The model under review builds one solid part; all positions refer to its coordinate system, in mm. A direction names the side the tool comes from. Coordinates: 2 decimals unless noted, no trailing zeros. Write each loop counter-clockwise with the first axis right and the second up, starting at its lowest first coordinate (ties: lowest second). Pieces come first, ordered by that corner, then holes. Notation, with made-up numbers: (6.5, 49.5) - (22.5, 49.5) arc R9 cw to (22.5, 62.5) - close; hole circle Ø4 at (9, 24.25). An arc over 180 degrees is marked (long way). Use one line per item in the form item = value. Start each with the question number.
```python
from build123d import *
from OCP.BRepFilletAPI import BRepFilletAPI_MakeFillet

# Parameters (mm, degrees)
SKETCH_1_R      = 1.54
EXTRUDE_1_DEPTH = 5
SKETCH_2_R      = 1.7
EXTRUDE_2_DEPTH = 5
FILLET_1_R1     = 3
FILLET_1_R2     = 8


with BuildPart() as part:
    # 草图1 → 凸台-拉伸1 (new body)
    with BuildSketch(Plane.XY):
        with BuildLine():
            Line((0, -28.5), (76.583465403, -28.5))
            Line((76.583465403, -28.5), (76.583465403, 28.5))
            Line((76.583465403, 28.5), (0, 28.5))
            ThreePointArc((0, 28.5), (-28.5, 0), (0, -28.5))
        make_face()
        with Locations((-13.5, 0)):
            Circle(SKETCH_1_R, mode=Mode.SUBTRACT)
        with Locations((6.75, 11.691342951)):
            Circle(SKETCH_1_R, mode=Mode.SUBTRACT)
        with Locations((6.75, -11.691342951)):
            Circle(SKETCH_1_R, mode=Mode.SUBTRACT)
    extrude(amount=EXTRUDE_1_DEPTH)

    # 草图2 → 凸台-拉伸2 (add)
    with BuildSketch(Plane(origin=(76.583465403, 0, 0), x_dir=(0, 0, -1), z_dir=(1, 0, 0))):
        with BuildLine():
            Line((0, -28.5), (0, 28.5))
            Line((0, 28.5), (-60, 28.5))
            ThreePointArc((-60, 28.5), (-88.5, 0), (-60, -28.5))
            Line((-60, -28.5), (0, -28.5))
        make_face()
        with Locations((-73.435028843, -13.435028843)):
            Circle(SKETCH_2_R, mode=Mode.SUBTRACT)
        with Locations((-73.435028843, 13.435028843)):
            Circle(SKETCH_2_R, mode=Mode.SUBTRACT)
        with Locations((-46.564971157, 13.435028843)):
            Circle(SKETCH_2_R, mode=Mode.SUBTRACT)
        with Locations((-46.564971157, -13.435028843)):
            Circle(SKETCH_2_R, mode=Mode.SUBTRACT)
    extrude(amount=EXTRUDE_2_DEPTH)

    # 圆角1: one fillet with a radius per group of edges: ONE call of the kernel's fillet builder (fillet() takes one radius for all edges)
    fillet_1_edges_1 = [part.edges().sort_by_distance(p)[0] for p in [
        (76.583465403, 0, 5),
    ]]
    fillet_1_edges_2 = [part.edges().sort_by_distance(p)[0] for p in [
        (81.583465403, 0, 0),
    ]]
    fillet_1 = BRepFilletAPI_MakeFillet(part.part.solid().wrapped)
    for e in fillet_1_edges_1:
        fillet_1.Add(FILLET_1_R1, e.wrapped)
    for e in fillet_1_edges_2:
        fillet_1.Add(FILLET_1_R2, e.wrapped)
    add(Compound.cast(fillet_1.Shape()), mode=Mode.REPLACE)


solid = part.part
```
1. Take a section at C-C (y = 18.5). State the section outline as (x, z) points.
2. For faces 4 (the flat face through (76.583, 0, 49)), 5 (the flat face through (59, -28.5, 3)), list the 3-axis set-ups (+Z, -Z, +X, -X, +Y, -Y) from which the entire face can be reached by the end or side of a thin tool; tool diameter is ignored.
3. For P1, Ø8, axis at x = 31, z = 12.5, coming from the +Y side; P2, Ø5.5, axis at y = -13.44, z = 46.56, coming from the -X side; P3, Ø6, axis at x = -6.5, y = 13.5, coming from the +Z side, all flat-tipped, find the tip position at first contact; note any pin that passes through.
4. The part is to be moulded in two halves that separate along X. For faces 1 (the cylindrical face through (5.615, 12.732, 2.465)), 2 (the cylindrical face through (79.048, 0.627, 88.493)), 3 (the cylindrical face through (-28.493, 0.627, 2.465)), say which applies: released by +X, released by -X, zero draft, split by the parting line, or undercut.
5. Take a section at A-A (y = 0). State the section outline as (x, z) points.
6. Take a section at D-D (x = 53). State the section outline as (y, z) points, plus the area to 3 significant figures.
7. Take a section at B-B (x = 6.75). State the section outline as (y, z) points.
8. For L1, parallel to Z at x = 39, y = 14; L2, parallel to Y at x = -13.5, z = 3.05; L3, parallel to X at y = 5, z = 72.5, list the stretches that pass through material, from the lowest coordinate up.
Returned:
q1.outline = (-21.68, 0) - (73.58, 0) arc R8 ccw to (81.58, 8) - (81.58, 81.68) - (76.58, 81.68) - (76.58, 8) arc R3 cw to (73.58, 5) - (-21.68, 5) - close
q2.face_4 = +Z, -X, +Y, -Y
q2.face_5 = +Z, -Z, +X, -X, -Y
q3.P1 = through
q3.P2 = 76.58
q3.P3 = 5
q4.face_1 = undercut
q4.face_2 = zero draft
q4.face_3 = released by -X
q5.outline = (-28.5, 0) - (-15.04, 0) - (-15.04, 5) - (-28.5, 5) - close; (-11.96, 0) - (73.58, 0) arc R8 ccw to (81.58, 8) - (81.58, 88.5) - (76.58, 88.5) - (76.58, 8) arc R3 cw to (73.58, 5) - (-11.96, 5) - close
q6.outline = (-28.5, 0) - (28.5, 0) - (28.5, 5) - (-28.5, 5) - close
q6.area = 285 mm²
q7.outline = (-28.5, 0) - (-13.23, 0) - (-13.23, 5) - (-28.5, 5) - close; (-10.15, 0) - (10.15, 0) - (10.15, 5) - (-10.15, 5) - close; (13.23, 0) - (28.5, 0) - (28.5, 5) - (13.23, 5) - close
q8.L1 = 0 to 5
q8.L2 = -25.1 to -1.54, 1.54 to 25.1
q8.L3 = 76.58 to 81.58
